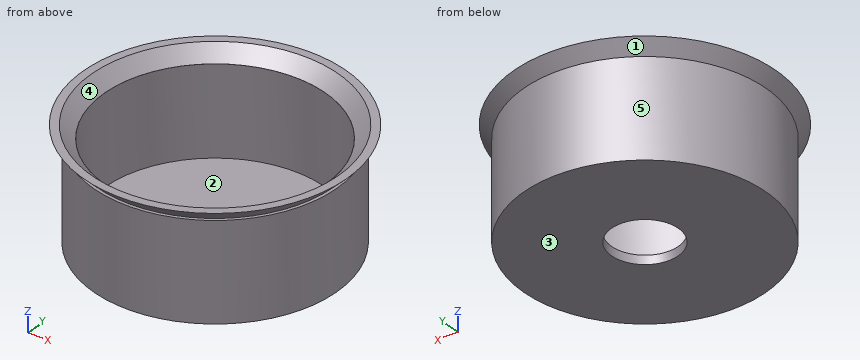
```python
from build123d import *

# Parameters (mm, degrees)
SKETCH125_R     = 34.925
PAD046_DEPTH    = 27.94
SKETCH126_R     = 31.75
POCKET046_DEPTH = 25.4
SKETCH127_R     = 9.6139
POCKET047_DEPTH = 27.941


with BuildPart() as part:
    # Sketch125 → Pad046 (new body)
    with BuildSketch(Plane.XY):
        Circle(SKETCH125_R)
    extrude(amount=PAD046_DEPTH)

    # Sketch126 (on Face3 of Pad046) → Pocket046 (cut)
    with BuildSketch(Plane.XY.offset(27.94)):
        Circle(SKETCH126_R)
    extrude(amount=-POCKET046_DEPTH, mode=Mode.SUBTRACT)

    # Sketch127 (on Face2 of Pocket046) → Pocket047 (cut, through all)
    with BuildSketch(Plane(origin=(0, 0, 0), x_dir=(1, 0, 0), z_dir=(0, 0, -1))):
        Circle(SKETCH127_R)
    extrude(amount=-POCKET047_DEPTH, mode=Mode.SUBTRACT)

    # Sketch131 → Revolution001 (revolve)
    with BuildSketch(Plane.XZ):
        Polygon((34.041662, 27.921203), (37.778515, 31.658056), (35.500414, 31.658056), (31.763561, 27.921203), align=None)
    revolve(axis=Axis((0, 0, 0), (0, 0, 1)))


solid = part.part
```
Input: part model. Units: mm. Frame: model coordinates. Face numbers are marked on the shaded views. A direction names the side the tool comes from. Give positions to 0.01 mm unless a question says otherwise; leave off trailing zeros. Order: outer loops, then holes, each group sorted by start corner. A loop starts at its lowest first (then second) coordinate and runs counter-clockwise, first axis right, second up.
1. Set-up query: the marked faces 1 and 2. Return all of +Z, -Z, +X, -X, +Y, -Y with unobstructed straight access to the full face (end or side cutting, diameter ignored); none if empty.
Computed:
face 1: none
face 2: +Z
2. Pin query (flat end, axial travel): pin 1 Ø2 at (x, z) = (23, 12.5) entering from -Y; pin 2 Ø4 at (x, z) = (27.5, 28) entering from +Y; pin 3 Ø10 at (x, y) = (4.5, -18.5) entering from -Z; pin 4 Ø10 at (y, z) = (-1.5, 23) entering from +X (3 decimals). Return the tip coordinate at first contact, or that it passes through.
Computed:
pin 1: stops at y = -27.12
pin 2: stops at y = 24.17
pin 3: stops at z = 0
pin 4: stops at x = 34.925
3. Draft query along Y for the marked faces 3, 4 and 5. Return one class per face: released by +Y, released by -Y, zero draft, split by the parting line, or undercut.
Computed:
face 3: zero draft
face 4: undercut
face 5: split by the parting line
4. Cut plane A-A (x = 0). Return loops of the section in (y, z) (3 decimals).
Computed:
outline: (-37.779, 31.658) - (-34.06, 27.94) - (-34.925, 27.94) - (-34.925, 0) - (-9.614, 0) - (-9.614, 2.54) - (-31.75, 2.54) - (-31.75, 27.94) - (-31.782, 27.94) - (-35.5, 31.658) - close; (9.614, 0) - (34.925, 0) - (34.925, 27.94) - (34.06, 27.94) - (37.779, 31.658) - (35.5, 31.658) - (31.782, 27.94) - (31.75, 27.94) - (31.75, 2.54) - (9.614, 2.54) - close
5. Line query: probe 1 along Y at (x, z) = (0, 8.5) (3 decimals); probe 2 along Y at (x, z) = (0, 0.65) (3 decimals); probe 3 along Z at (x, y) = (-4, -20). Output: solid intervals per line, ascending.
Computed:
probe 1: y = -34.925 to -31.75, 31.75 to 34.925
probe 2: y = -34.925 to -9.614, 9.614 to 34.925
probe 3: z = 0 to 2.54
6. Cut plane C-C (z = 19). Return loops of the section in (x, y) (3 decimals), and give its area (3 significant figures).
Computed:
outline: circle Ø69.85 at (0, 0); hole circle Ø63.5 at (0, 0)
area: 665 mm2
